Verification items for this drawing (mm, ordinates from the low corner). A direction names the side the tool comes from. Coordinates: 2 decimals unless noted, no trailing zeros. Order: outer loops, then holes, each group sorted by start corner. A loop starts at its lowest first (then second) coordinate and runs counter-clockwise, first axis right, second up.
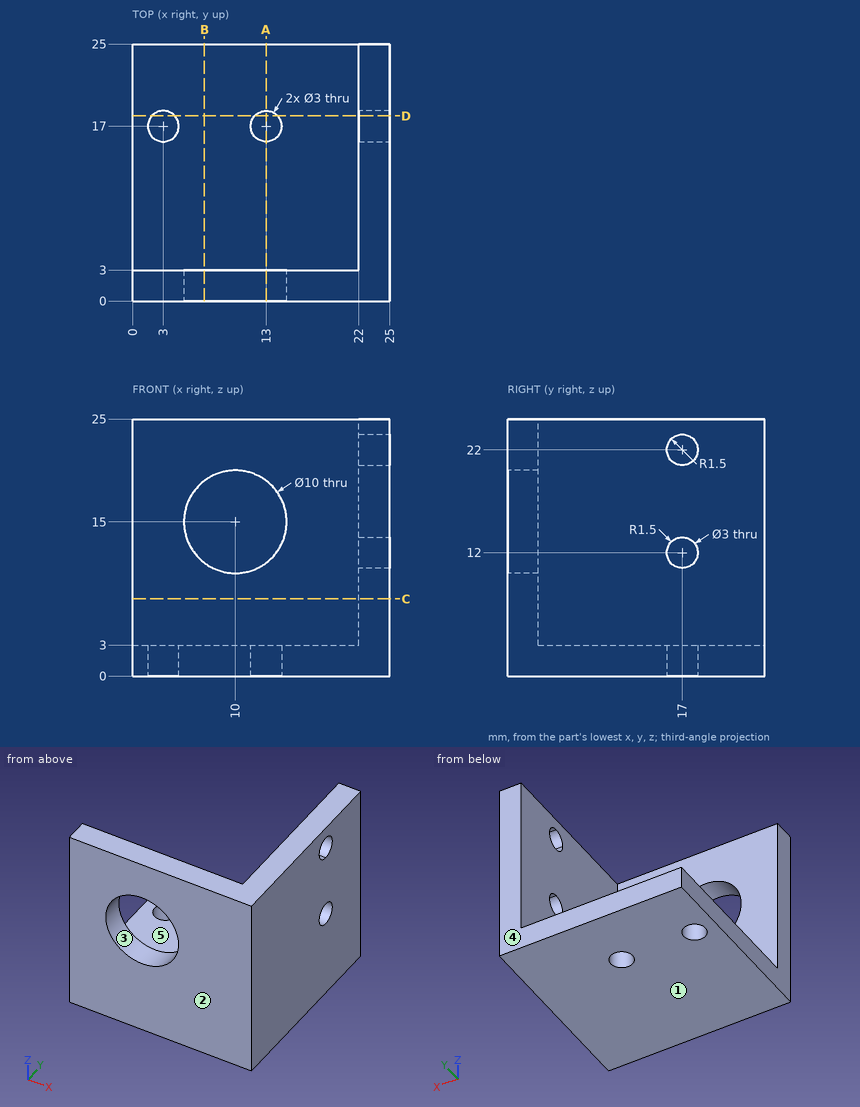
(1) Tool access check on the marked faces 4 and 5. Record the directions out of +Z, -Z, +X, -X, +Y, -Y that give a thin tool (end or side, any length) a straight path to the whole face; none if there is none.
Filled in:
face 4: +Z, -Z, +X, -X, +Y
face 5: +Z, -X, +Y
(2) Cross-section at A-A (x = 13). Enter the section's corners in (y, z).
Filled in:
outline: (0, 0) - (15.5, 0) - (15.5, 3) - (3, 3) - (3, 11) - (0, 11) - close; (0, 19) - (3, 19) - (3, 25) - (0, 25) - close; (18.5, 0) - (25, 0) - (25, 3) - (18.5, 3) - close
(3) Go/stop test with flat-tipped pins: P1, Ø1, axis at x = 11.5, y = 5.5, coming from the +Z side; P2, Ø5, axis at y = 17, z = 12, coming from the +X side; P3, Ø11, axis at x = 8, z = 17.5, coming from the +Y side; P4, Ø6, axis at y = 7, z = 13, coming from the -X side. Record where each tip stops, or that it passes through.
Filled in:
P1: stops at z = 3
P2: stops at x = 25
P3: stops at y = 3
P4: stops at x = 22
(4) Cross-section at B-B (x = 7). Enter the section's corners in (y, z).
Filled in:
outline: (0, 0) - (25, 0) - (25, 3) - (3, 3) - (3, 11) - (0, 11) - close; (0, 19) - (3, 19) - (3, 25) - (0, 25) - close
(5) Cross-section at C-C (z = 7.5). Enter the section's corners in (x, y), and give its area (3 significant figures).
Filled in:
outline: (0, 0) - (25, 0) - (25, 25) - (22, 25) - (22, 3) - (0, 3) - close
area: 141 mm2
(6) Release check for a two-part mould opening along Z. For the marked faces 1, 2 and 3 record: +Z half, -Z half, draft (parallel to the pull), parting line (faces both ways), or undercut.
Filled in:
face 1: -Z half
face 2: draft
face 3: undercut
(7) Cross-section at D-D (y = 18). Enter the section's corners in (x, z), and give its area (3 significant figures).
Filled in:
outline: (0, 0) - (1.88, 0) - (1.88, 3) - (0, 3) - close; (4.12, 0) - (11.88, 0) - (11.88, 3) - (4.12, 3) - close; (14.12, 0) - (25, 0) - (25, 10.88) - (22, 10.88) - (22, 3) - (14.12, 3) - close; (22, 13.12) - (25, 13.12) - (25, 20.88) - (22, 20.88) - close; (22, 23.12) - (25, 23.12) - (25, 25) - (22, 25) - close
area: 114 mm2
(8) Thickness scan on probe 1 along Z at (x, y) = (23.9, 17); probe 2 along Y at (x, z) = (13, 1.95); probe 3 along Z at (x, y) = (21.25, 9.75). Record the ranges inside material, lowest first.
Filled in:
probe 1: z = 0 to 10.5, 13.5 to 20.5, 23.5 to 25
probe 2: y = 0 to 15.5, 18.5 to 25
probe 3: z = 0 to 3
